Input: part model. Units: mm. Frame: model coordinates. Face numbers are marked on the shaded views. A direction names the side the tool comes from. Round coordinates to 2 decimals unless told otherwise and drop trailing zeros. Order: outer loops, then holes, each group sorted by start corner. A loop starts at its lowest first (then second) coordinate and runs counter-clockwise, first axis right, second up.
Item 1: First-contact query: pin 1 (3 mm diameter, centred on x = 9, y = 0, fed in from -Z); pin 2 (1.5 mm diameter, centred on x = 5, z = 10, fed in from -Y); pin 3 (3 mm diameter, centred on y = -5, z = 9, fed in from -X); pin 4 (1 mm diameter, centred on x = 14.5, z = 3.5, fed in from +Y). Flat tips, straight axial feed; report the tip coordinate or a pass-through.
Item 2: Cut plane B-B on x = -11. Output: boundary loops of the cut face in (y, z).
Item 3: Reachability of the marked faces 1 and 2 from +Z, -Z, +X, -X, +Y, -Y: full face, straight path, thin tool, end or side. Return the list, or none.
Item 4: Cut plane C-C on z = 11.75. Output: boundary loops of the cut face in (x, y).
Item 5: Cut plane D-D on y = -17.5. Output: boundary loops of the cut face in (x, z), then the cut area to 3 significant figures.
Item 6: Mould query, pull axis Y, two halves, no side actions, for the marked faces 3, 4, 5 and 6. Classes: released by +Y, released by -Y, zero draft, split by the parting line, or undercut.
Item 7: Line query: L1, parallel to X at y = -10.75, z = 7; L2, parallel to Y at x = -16.5, z = 7.75; L3, parallel to Z at x = -12, y = -10.25. Output: solid intervals per line, ascending.
Item 8: Cut plane A-A on y = 0. Output: boundary loops of the cut face in (x, z), then the cut area to 3 significant figures.
```python
from build123d import *

# Parameters (mm, degrees)
PAD_DEPTH            = 14
POCKET_DEPTH         = 6
SKETCH002_R          = 2.25
POCKET001_DEPTH      = 46.001
SKETCH003_R          = 2.339712
POCKET002_DEPTH      = 1000
POCKET002_DEPTH_BACK = -100
FILLET_R             = 2.88


with BuildPart() as part:
    # Sketch → Pad (new body)
    with BuildSketch(Plane.XY):
        Polygon((-22, 7), (6, 7), (6, -7), (-22, -7), (-22, -22), (0, -22), (24, -13), (24, 13), (0, 22), (-22, 22), align=None)
    extrude(amount=PAD_DEPTH)

    # Sketch001 (on Face2 of Pad) → Pocket (cut)
    with BuildSketch(Plane(origin=(6, 0, 0), x_dir=(0, -1, 0), z_dir=(-1, 0, 0))):
        Polygon((-2.020726, 3.5), (2.020726, 3.5), (4.041452, 7), (2.020726, 10.5), (-2.020726, 10.5), (-4.041452, 7), align=None)
    extrude(amount=-POCKET_DEPTH, mode=Mode.SUBTRACT)

    # Sketch002 (on Face17 of Pocket) → Pocket001 (cut, through all)
    with BuildSketch(Plane.YZ.offset(24)):
        with Locations((0, 7)):
            Circle(SKETCH002_R)
    extrude(amount=-POCKET001_DEPTH, mode=Mode.SUBTRACT)

    # Sketch003 (on Face1 of Pocket001) → Pocket002 (cut, two sides)
    with BuildSketch(Plane.XZ.offset(-7)) as pocket002_sk:
        with Locations((-12, 7)):
            Circle(SKETCH003_R)
    extrude(amount=-POCKET002_DEPTH, mode=Mode.SUBTRACT)
    extrude(pocket002_sk.sketch, amount=-POCKET002_DEPTH_BACK, mode=Mode.SUBTRACT)

    # Fillet
    fillet_edges = [part.edges().sort_by_distance(p)[0] for p in [
        (6, -7, 7),
        (6, 7, 7),
        (-22, -7, 7),
        (-22, -22, 7),
        (0, -22, 7),
        (24, -13, 7),
        (24, 13, 7),
        (0, 22, 7),
        (-22, 22, 7),
        (-22, 7, 7),
    ]]
    fillet(fillet_edges, radius=FILLET_R)


solid = part.part
```
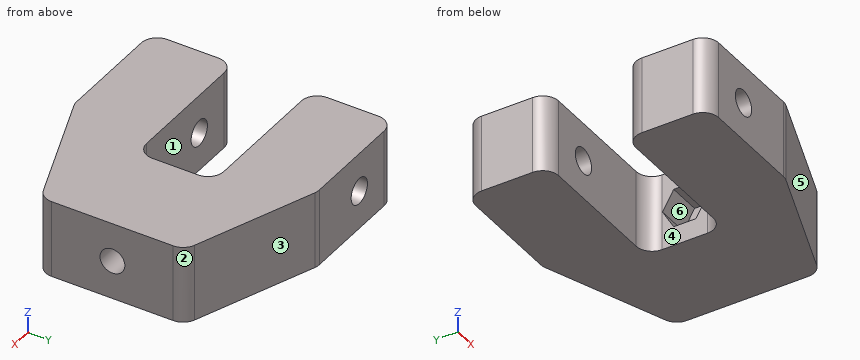
From the geometry:
1. pin 1: stops at z = 0
1. pin 2: stops at y = -20.41
1. pin 3: stops at x = 4.74
1. pin 4: stops at y = 16.75
2. outline: (-22, 0) - (-7, 0) - (-7, 4.88) - (-22, 4.88) - close; (-22, 9.12) - (-7, 9.12) - (-7, 14) - (-22, 14) - close; (7, 0) - (22, 0) - (22, 4.88) - (7, 4.88) - close; (7, 9.12) - (22, 9.12) - (22, 14) - (7, 14) - close
3. face 1: +Z, -Z, -X
3. face 2: +Z, -Z, +X, +Y
4. outline: (-22, -19.12) arc R2.88 ccw to (-19.12, -22) - (-0.52, -22) arc R2.88 ccw to (0.49, -21.82) - (22.13, -13.7) arc R2.88 ccw to (24, -11) - (24, 11) arc R2.88 ccw to (22.13, 13.7) - (0.49, 21.82) arc R2.88 ccw to (-0.52, 22) - (-19.12, 22) arc R2.88 ccw to (-22, 19.12) - (-22, 9.88) arc R2.88 ccw to (-19.12, 7) - (3.12, 7) arc R2.88 cw to (6, 4.12) - (6, -4.12) arc R2.88 cw to (3.12, -7) - (-19.12, -7) arc R2.88 ccw to (-22, -9.88) - close
5. outline: (-22, 0) - (12, 0) - (12, 14) - (-22, 14) - close; hole circle Ø4.68 at (-12, 7)
5. area: 459 mm2
6. face 3: released by +Y
6. face 4: undercut
6. face 5: released by -Y
6. face 6: undercut
7. L1: x = -22 to -14.34, -9.66 to 24
7. L2: y = -22 to -7, 7 to 22
7. L3: z = 0 to 4.66, 9.34 to 14
8. outline: (6, 0) - (24, 0) - (24, 4.75) - (12, 4.75) - (12, 3.5) - (6, 3.5) - close; (6, 10.5) - (12, 10.5) - (12, 9.25) - (24, 9.25) - (24, 14) - (6, 14) - close
8. area: 156 mm2
